Part print with two shaded views. Sizes in mm from the minimum x, y, z corner. Give positions to 0.01 mm unless a question says otherwise; leave off trailing zeros. Write each loop counter-clockwise with the first axis right and the second up, starting at its lowest first coordinate (ties: lowest second). Pieces come first, ordered by that corner, then holes.
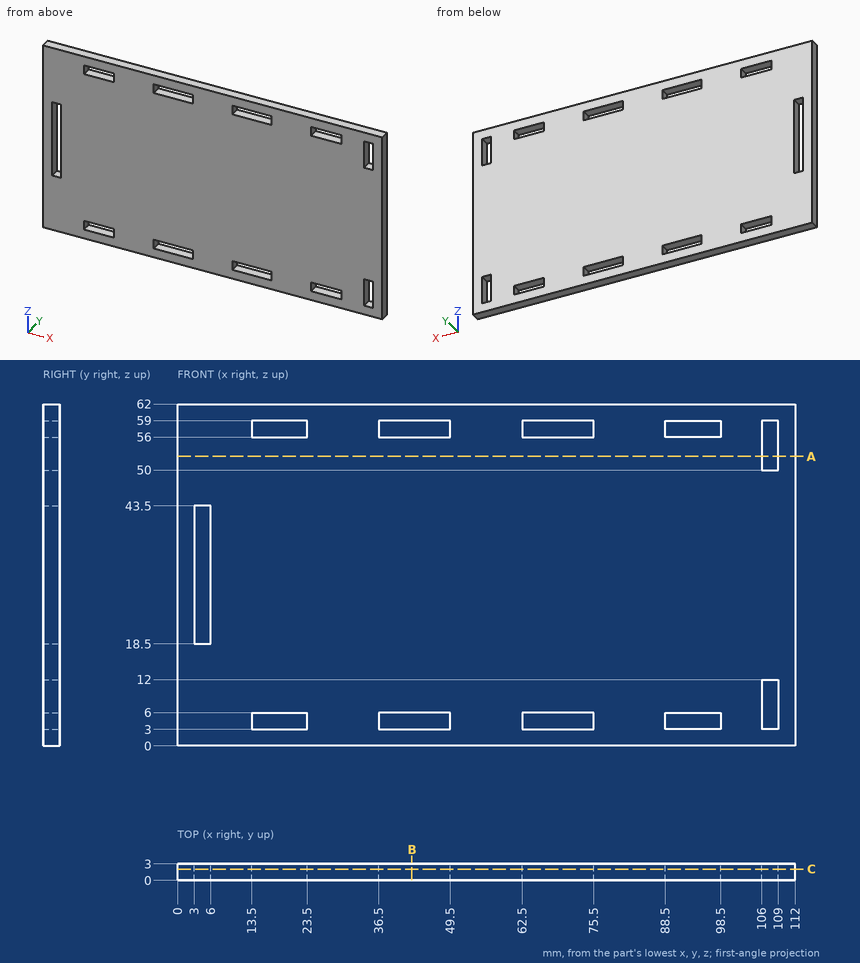
1) Wall check: L1, parallel to Z at x = 19.5, y = 2.9; L2, parallel to X at y = 2.5, z = 42; L3, parallel to X at y = 1.2, z = 10. Give the ranges that are in metal, low to high.
Answers follow:
L1: z = 0 to 3, 6 to 56, 59 to 62
L2: x = 0 to 3, 6 to 112
L3: x = 0 to 106, 109 to 112
2) Pin check, flat tip, straight feed: pin 1 Ø3 at (x, z) = (41.5, 44) entering from -Y. Stop position of the tip, or through.
Answers follow:
pin 1: stops at y = 0
3) Saw through at C-C, the plane y = 2.05. Count the separate pieces of the cut face and the enclosed holes in it, then the cut area to 3 significant figures.
Answers follow:
separate pieces: 1
enclosed holes: 11
area: 6,540 mm2
4) Saw through at A-A, the plane z = 52.5. Write the cut outline in (x, y).
Answers follow:
outline: (0, 0) - (106, 0) - (106, 3) - (0, 3) - close; (109, 0) - (112, 0) - (112, 3) - (109, 3) - close
5) Saw through at B-B, the plane x = 42.5. Write the cut outline in (y, z), then the cut area to 3 significant figures.
Answers follow:
outline: (0, 0) - (3, 0) - (3, 3) - (0, 3) - close; (0, 6) - (3, 6) - (3, 56) - (0, 56) - close; (0, 59) - (3, 59) - (3, 62) - (0, 62) - close
area: 168 mm2
